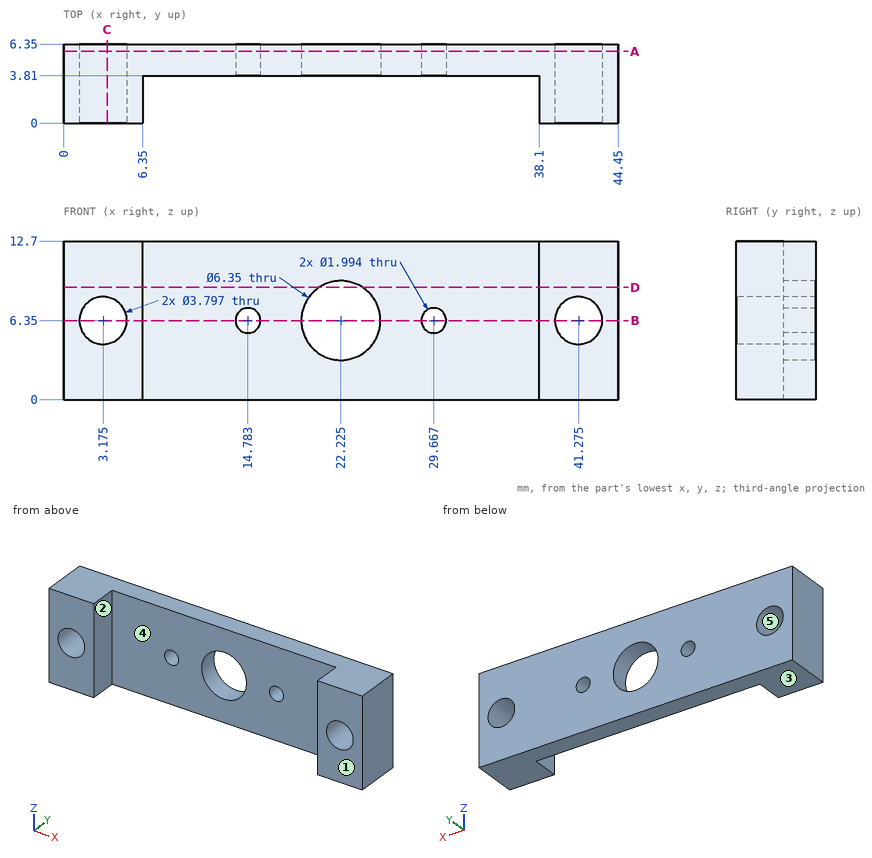
For this review, use the dimensioned drawing (mm, ordinates from the lowest corner) and the shaded views. A direction names the side the tool comes from. Give positions to 0.01 mm unless a question says otherwise; leave off trailing zeros. Order: outer loops, then holes, each group sorted by start corner. A loop starts at its lowest first (then second) coordinate and runs counter-clockwise, first axis right, second up. Notation, with made-up numbers: (7.5, 29.5) - (29.5, 29.5) arc R10 ccw to (29.5, 39.5) - close; hole circle Ø11 at (26, 38). An arc over 180 degrees is marked (long way). Write item = value, one per line. Start each with the question number.
Q1. Mouldability with a two-part tool opening along Z and no side actions: class the marked faces 3, 4 and 5 as released by +Z, released by -Z, zero draft, split by the parting line, or undercut.
Q2. To check wall thickness, follow L1, parallel to X at y = 0.5, z = 2; L2, parallel to X at y = 5.5, z = 7; L3, parallel to Y at x = 23, z = 2. State the ranges of each line that lie inside material, in increasing order. Write a range as from..to.
Q3. We need section C-C on x = 3.5. State the section outline as (y, z) points, plus the area to 3 significant figures.
Q4. We need section B-B on z = 6.35. State the section outline as (x, y) points.
Q5. We need section D-D on z = 9. State the section outline as (x, y) points, plus the area to 3 significant figures.
Q6. We need section A-A on y = 5.75. State how many separate pieces and enclosed holes the cut face has, plus the area to 3 significant figures.
Q7. Clearance check with flat-ended pins moving along their axes: pin 1 Ø4 at (x, z) = (22.225, 6.35) entering from -Y; pin 2 Ø3 at (x, z) = (14.78, 6.35) entering from -Y. State where each tip first meets the part, or that it passes through.
Q8. Tool access review of the marked faces 1 and 2: name each direction out of +Z, -Z, +X, -X, +Y, -Y from which nothing blocks a thin tool from reaching the whole face with its end or side.
Working result:
q1.face_3 = released by -Z
q1.face_4 = zero draft
q1.face_5 = undercut
q2.L1 = 0..6.35, 38.1..44.45
q2.L2 = 0..1.39, 4.96..14.03, 15.54..19.12, 25.33..28.91, 30.42..39.49, 43.06..44.45
q2.L3 = 3.81..6.35
q3.outline = (0, 0) - (6.35, 0) - (6.35, 4.48) - (0, 4.48) - close; (0, 8.22) - (6.35, 8.22) - (6.35, 12.7) - (0, 12.7) - close
q3.area = 56.9 mm²
q4.outline = (0, 0) - (1.28, 0) - (1.28, 6.35) - (0, 6.35) - close; (5.07, 0) - (6.35, 0) - (6.35, 3.81) - (13.79, 3.81) - (13.79, 6.35) - (5.07, 6.35) - close; (15.78, 3.81) - (19.05, 3.81) - (19.05, 6.35) - (15.78, 6.35) - close; (25.4, 3.81) - (28.67, 3.81) - (28.67, 6.35) - (25.4, 6.35) - close; (30.66, 3.81) - (38.1, 3.81) - (38.1, 0) - (39.38, 0) - (39.38, 6.35) - (30.66, 6.35) - close; (43.17, 0) - (44.45, 0) - (44.45, 6.35) - (43.17, 6.35) - close
q5.outline = (0, 0) - (6.35, 0) - (6.35, 3.81) - (20.48, 3.81) - (20.48, 6.35) - (0, 6.35) - close; (23.97, 3.81) - (38.1, 3.81) - (38.1, 0) - (44.45, 0) - (44.45, 6.35) - (23.97, 6.35) - close
q5.area = 152 mm²
q6.separate_pieces = 1
q6.enclosed_holes = 5
q6.area = 504 mm²
q7.pin_1 = through
q7.pin_2 = 3.81
q8.face_1 = +Z, -Z, +X, -X, -Y
q8.face_2 = +Z, -Z, -Y
